```python
from build123d import *

# Parameters (mm, degrees)
SKETCH007_W      = 27.27
SKETCH007_H      = 19.5
SKETCH007_W_2    = 9
SKETCH007_H_2    = 1.75
EXTRUDE006_DEPTH = 2
SKETCH006_W      = 27.27
SKETCH006_H      = 27.31
SKETCH006_R      = 0.25
EXTRUDE007_DEPTH = 1
SKETCH008_W      = 10.4
SKETCH008_H      = 2.5
EXTRUDE008_DEPTH = 8.5
SKETCH009_W      = 10.4
SKETCH009_H      = 2.5
EXTRUDE009_DEPTH = 21.5


with BuildPart() as obj1:
    # Sketch007 → Extrude006 (new body)
    with BuildSketch(Plane.XY):
        with Locations((13.635, 13.36)):
            Rectangle(SKETCH007_W, SKETCH007_H)
        with Locations((13.635, 25.435)):
            Rectangle(SKETCH007_W_2, SKETCH007_H_2)
    extrude(amount=EXTRUDE006_DEPTH)


with BuildPart() as obj1_1:
    # Extrude006 placement: moved
    add(obj1.part.moved(Location((0, 0, 1))))


with BuildPart() as extrude_display_base:
    # Sketch006 → Extrude007 (new body)
    with BuildSketch(Plane.XY):
        with Locations((13.635, 13.655)):
            Rectangle(SKETCH006_W, SKETCH006_H)
        with Locations((8.514, 25.135)):
            Circle(SKETCH006_R, mode=Mode.SUBTRACT)
        with Locations((11.928, 25.135)):
            Circle(SKETCH006_R, mode=Mode.SUBTRACT)
        with Locations((15.342, 25.135)):
            Circle(SKETCH006_R, mode=Mode.SUBTRACT)
        with Locations((18.756, 25.135)):
            Circle(SKETCH006_R, mode=Mode.SUBTRACT)
        with BuildLine():
            ThreePointArc((2.775, 26.31), (1.6, 25.135), (2.775, 23.96))
            Line((2.775, 23.96), (3.925, 23.96))
            ThreePointArc((3.925, 23.96), (5.1, 25.135), (3.925, 26.31))
            Line((3.925, 26.31), (2.775, 26.31))
        make_face(mode=Mode.SUBTRACT)
        with BuildLine():
            ThreePointArc((23.345, 26.31), (22.17, 25.135), (23.345, 23.96))
            Line((23.345, 23.96), (24.495, 23.96))
            ThreePointArc((24.495, 23.96), (25.67, 25.135), (24.495, 26.31))
            Line((24.495, 26.31), (23.345, 26.31))
        make_face(mode=Mode.SUBTRACT)
        with BuildLine():
            ThreePointArc((2.775, 3.1), (1.6, 1.925), (2.775, 0.75))
            Line((2.775, 0.75), (3.925, 0.75))
            ThreePointArc((3.925, 0.75), (5.1, 1.925), (3.925, 3.1))
            Line((3.925, 3.1), (2.775, 3.1))
        make_face(mode=Mode.SUBTRACT)
        with BuildLine():
            ThreePointArc((23.345, 3.1), (22.17, 1.925), (23.345, 0.75))
            Line((23.345, 0.75), (24.495, 0.75))
            ThreePointArc((24.495, 0.75), (25.67, 1.925), (24.495, 3.1))
            Line((24.495, 3.1), (23.345, 3.1))
        make_face(mode=Mode.SUBTRACT)
    extrude(amount=EXTRUDE007_DEPTH)


with BuildPart() as fusion_display:
    # Sketch008 → Extrude008 (new body)
    with BuildSketch(Plane.XY):
        with Locations((13.635, 25.36)):
            Rectangle(SKETCH008_W, SKETCH008_H)
    extrude(amount=-EXTRUDE008_DEPTH)

    # Fusion002: union obj1, Extrude_Display_base
    add(obj1_1.part)
    add(extrude_display_base.part)


with BuildPart() as obj2:
    # Sketch009 → Extrude009 (new body)
    with BuildSketch(Plane.XY):
        with Locations((13.635, 25.36)):
            Rectangle(SKETCH009_W, SKETCH009_H)
    extrude(amount=-EXTRUDE009_DEPTH)

    # Fusion003: union Fusion_Display
    add(fusion_display.part)


with BuildPart() as obj2_1:
    # Fusion003 placement: moved
    add(obj2.part.moved(Location((-50, 0, 0))))


solid = obj2_1.part
```
Geometry: final body of the model. Coordinates: model frame, mm. A direction names the side the tool comes from. Round coordinates to 2 decimals unless told otherwise and drop trailing zeros. Order: outer loops, then holes, each group sorted by start corner. A loop starts at its lowest first (then second) coordinate and runs counter-clockwise, first axis right, second up. Notation, with made-up numbers: M 47,3 L 86,3 A26 cw 86,19 Z; hole C -2.75,-36.75 d9. An arc over 180 degrees is marked long. Use one line per item in the form item = value. Start each with the question number.
Q1. Pin query (flat end, axial travel): pin 1 Ø3 at (x, z) = (-36.5, -10.5) entering from -Y; pin 2 Ø3 at (x, z) = (-38.5, -8.5) entering from +Y; pin 3 Ø2 at (y, z) = (25.5, -11) entering from +X (3 decimals); pin 4 Ø12 at (y, z) = (5.5, -0.5) entering from -X. Return the tip coordinate at first contact, or that it passes through.
Q2. Cut plane A-A (x = -48). Return loops of the section in (y, z).
Q3. Cut plane B-B (x = -44). Return loops of the section in (y, z).
Q4. Material intervals for line 1 (Y direction, x = -41, z = -5.5); line 2 (Z direction, x = -35, y = 21); line 3 (Y direction, x = -36.25, z = 1.5), sorted ascending. Write a range as [from, to].
Q5. Access query for faces 5 (the face through (-37, 2, 1)), 6 (the face through (-36.6, 0, 0.5)), 7 (the face through (-36, 25, 3)), 8 (the face through (-36, 24.56, 2)), 9 (the face through (-26.1, 0.75, 0.5)). Directions: +Z, -Z, +X, -X, +Y, -Y. A direction counts if a zero-diameter tool reaches every point of the face in a straight line with its end or side. Return the directions, or none.
Q6. Mould query, pull axis Y, two halves, no side actions, for faces 1 (the face through (-37, 3.61, 2)), 2 (the face through (-27.83, 1.95, 0.49)), 3 (the face through (-36, 26.31, 2)), 4 (the face through (-31.165, 25, -11)). Classes: +Y half, -Y half, draft (parallel to the pull), parting line (faces both ways), or undercut.
Q7. Cut plane D-D (z = -1.5). Return loops of the section in (x, y) (3 decimals).
Q8. Cut plane C-C (y = 5.5). Return loops of the section in (x, z).
Geometry results:
q1.pin_1 = 24.11
q1.pin_2 = 26.61
q1.pin_3 = -31.165
q1.pin_4 = -50
q2.outline = M 0,0 L 1.04,0 L 1.04,1 L 0,1 Z; M 2.81,0 L 24.25,0 L 24.25,1 L 23.11,1 L 23.11,3 L 3.61,3 L 3.61,1 L 2.81,1 Z; M 26.02,0 L 27.31,0 L 27.31,1 L 26.02,1 Z
q3.outline = M 0,0 L 27.31,0 L 27.31,1 L 23.11,1 L 23.11,3 L 3.61,3 L 3.61,1 L 0,1 Z
q4.line_1 = [24.11, 26.61]
q4.line_2 = [0, 3]
q4.line_3 = [3.61, 23.11], [24.56, 26.31]
q5.face_5 = +Z, +X, -X, -Y
q5.face_6 = +Z, -Z, +X, -X, -Y
q5.face_7 = +Z, +X, -X, +Y, -Y
q5.face_8 = +Z, +X, -X
q5.face_9 = +Z, -Z
q6.face_1 = -Y half
q6.face_2 = undercut
q6.face_3 = +Y half
q6.face_4 = draft
q7.outline = M -41.565,24.11 L -31.165,24.11 L -31.165,26.61 L -41.565,26.61 Z
q8.outline = M -50,0 L -22.73,0 L -22.73,3 L -50,3 Z
